Check sheet for the modelled part. Datum: model origin and axes. Units: mm. A direction names the side the tool comes from. Round coordinates to 2 decimals unless told otherwise and drop trailing zeros. Loops run counter-clockwise (first coordinate to the right, second up) from the corner with the lowest first, then second, coordinate; pieces in that order, holes last. Notation, with made-up numbers: (-26.5, -21.75) - (-5.5, -21.75) arc R5 cw to (-5.5, -14.75) - close; hole circle Ø9 at (2.5, 68.5). An arc over 180 degrees is marked (long way). Return JSON: item names as keys, results as strings.
from build123d import *

# Parameters (mm, degrees)
SKETCH1_R                = 6.985
BLANK_DISK_DEPTH         = 2
GEAR_TOOTH_CUT_DEPTH     = 11.657412937
GEAR_START               = -2.000000064
GEAR_TEETH_REVOLVE_DEPTH = 4.000000128
SKETCH4_R                = 0.75
HUB_EXTRUDE_DEPTH        = 0.635
HEX_BORE_CUT_DEPTH       = 11.643895353
HEX_BORE_CUT_DEPTH_BACK  = 11.643895353


# Read off the part's stored shape, not the designer's step: GEAR TEETH REVOLVE
with BuildPart() as part:
    # Sketch1 → BLANK DISK (new, symmetric)
    with BuildSketch(Plane.XY):
        Circle(SKETCH1_R)
    extrude(amount=BLANK_DISK_DEPTH, both=True)

    # Sketch2 → GEAR TOOTH CUT (cut, through all)
    with BuildSketch(Plane.XY.offset(2.000000064)):
        with BuildLine():
            ThreePointArc((-5.763009467, -3.946890786), (-6.563752956, -2.389010701), (-6.951733872, -0.680897326))
            ThreePointArc((-6.951733872, -0.680897326), (-6.303106227, -0.89616004), (-5.627259472, -0.997585))
            ThreePointArc((-5.627259472, -0.997585), (-5.00805343, -1.01182167), (-4.389706578, -0.976241119))
            ThreePointArc((-4.389706578, -0.976241119), (-4.103194142, -1.046520353), (-3.923782009, -1.280699416))
            ThreePointArc((-3.923782009, -1.280699416), (-3.878581292, -1.411688142), (-3.82900912, -1.541085788))
            ThreePointArc((-3.82900912, -1.541085788), (-3.815919388, -1.835801253), (-3.990226026, -2.073804914))
            ThreePointArc((-3.990226026, -2.073804914), (-4.486777934, -2.444014326), (-4.951966126, -2.852938219))
            ThreePointArc((-4.951966126, -2.852938219), (-5.404500069, -3.365060167), (-5.763009467, -3.946890786))
        make_face()
    extrude(amount=-GEAR_TOOTH_CUT_DEPTH, mode=Mode.SUBTRACT)

    # GEAR TEETH REVOLVE outline → GEAR TEETH REVOLVE (cut)
    with BuildSketch(Plane.XY.offset(GEAR_START)):
        with BuildLine():
            ThreePointArc((-4.887664738, -4.990086011), (-3.4925, -6.049187445), (-1.877708884, -6.727884834))
            ThreePointArc((-1.877708884, -6.727884834), (-1.977068265, -6.051731323), (-1.959592795, -5.368539939))
            ThreePointArc((-1.959592795, -5.368539939), (-1.866089177, -4.756268856), (-1.723674371, -4.15349458))
            ThreePointArc((-1.723674371, -4.15349458), (-1.743133543, -3.859131051), (-1.942600309, -3.641779824))
            ThreePointArc((-1.942600309, -3.641779824), (-2.06375, -3.574519854), (-2.182573688, -3.503231129))
            ThreePointArc((-2.182573688, -3.503231129), (-2.470538755, -3.439163456), (-2.735194635, -3.569493083))
            ThreePointArc((-2.735194635, -3.569493083), (-3.186005068, -3.994215061), (-3.669495571, -4.381327111))
            ThreePointArc((-3.669495571, -4.381327111), (-4.25241893, -4.738057004), (-4.887664738, -4.990086011))
        make_face()
        with BuildLine():
            ThreePointArc((-0.536602953, -6.964357994), (1.212932521, -6.878882154), (2.886192555, -6.360826796))
            ThreePointArc((2.886192555, -6.360826796), (2.375455753, -5.906730136), (1.949695784, -5.372142157))
            ThreePointArc((1.949695784, -5.372142157), (1.627763445, -4.843012329), (1.34940368, -4.289717971))
            ThreePointArc((1.34940368, -4.289717971), (1.14528386, -4.07673054), (0.852772776, -4.038444607))
            ThreePointArc((0.852772776, -4.038444607), (0.716732854, -4.064794001), (0.579885119, -4.086562064))
            ThreePointArc((0.579885119, -4.086562064), (0.318109172, -4.222583755), (0.199145275, -4.492539562))
            ThreePointArc((0.199145275, -4.492539562), (0.126810473, -5.107670834), (0.00526609, -5.714997574))
            ThreePointArc((0.00526609, -5.714997574), (-0.211977555, -6.362964438), (-0.536602953, -6.964357994))
        make_face()
        with BuildLine():
            ThreePointArc((4.065541317, -5.67992947), (5.350820435, -4.489871453), (6.29961242, -3.017467208))
            ThreePointArc((6.29961242, -3.017467208), (5.616477625, -2.997904272), (4.946700037, -2.862059354))
            ThreePointArc((4.946700037, -2.862059354), (4.35996746, -2.663656509), (3.791080751, -2.418734649))
            ThreePointArc((3.791080751, -2.418734649), (3.497810216, -2.386782502), (3.249124002, -2.545476276))
            ThreePointArc((3.249124002, -2.545476276), (3.161848439, -2.653105859), (3.071009233, -2.757745191))
            ThreePointArc((3.071009233, -2.757745191), (2.957910282, -3.030210187), (3.040302898, -3.313476852))
            ThreePointArc((3.040302898, -3.313476852), (3.380289985, -3.831190659), (3.677563689, -4.374557157))
            ThreePointArc((3.677563689, -4.374557157), (3.927650474, -5.010570096), (4.065541317, -5.67992947))
        make_face()
        with BuildLine():
            ThreePointArc((6.765373622, -1.737798823), (6.985, 0), (6.765373622, 1.737798823))
            ThreePointArc((6.765373622, 1.737798823), (6.229487195, 1.313674319), (5.629088366, 0.987212828))
            ThreePointArc((5.629088366, 0.987212828), (5.052094245, 0.762053795), (4.458869006, 0.584001497))
            ThreePointArc((4.458869006, 0.584001497), (4.213672298, 0.419967595), (4.125173997, 0.138548695))
            ThreePointArc((4.125173997, 0.138548695), (4.1275, 0), (4.125173997, -0.138548695))
            ThreePointArc((4.125173997, -0.138548695), (4.213672298, -0.419967595), (4.458869006, -0.584001497))
            ThreePointArc((4.458869006, -0.584001497), (5.052094245, -0.762053795), (5.629088366, -0.987212828))
            ThreePointArc((5.629088366, -0.987212828), (6.229487195, -1.313674319), (6.765373622, -1.737798823))
        make_face()
        with BuildLine():
            ThreePointArc((6.29961242, 3.017467208), (5.350820435, 4.489871453), (4.065541318, 5.679929471))
            ThreePointArc((4.065541318, 5.679929471), (3.927650474, 5.010570096), (3.677563689, 4.374557157))
            ThreePointArc((3.677563689, 4.374557157), (3.380289985, 3.831190659), (3.040302898, 3.313476852))
            ThreePointArc((3.040302898, 3.313476852), (2.957910282, 3.030210187), (3.071009233, 2.757745191))
            ThreePointArc((3.071009233, 2.757745191), (3.161848439, 2.653105859), (3.249124002, 2.545476276))
            ThreePointArc((3.249124002, 2.545476276), (3.497810216, 2.386782502), (3.791080751, 2.418734649))
            ThreePointArc((3.791080751, 2.418734649), (4.35996746, 2.663656509), (4.946700037, 2.862059354))
            ThreePointArc((4.946700037, 2.862059354), (5.616477625, 2.997904272), (6.29961242, 3.017467208))
        make_face()
        with BuildLine():
            ThreePointArc((2.886192555, 6.360826797), (1.212932521, 6.878882155), (-0.536602953, 6.964357994))
            ThreePointArc((-0.536602953, 6.964357994), (-0.211977555, 6.362964438), (0.00526609, 5.714997574))
            ThreePointArc((0.00526609, 5.714997574), (0.126810473, 5.107670834), (0.199145275, 4.492539562))
            ThreePointArc((0.199145275, 4.492539562), (0.318109172, 4.222583755), (0.579885119, 4.086562064))
            ThreePointArc((0.579885119, 4.086562064), (0.716732854, 4.064794001), (0.852772776, 4.038444607))
            ThreePointArc((0.852772776, 4.038444607), (1.14528386, 4.07673054), (1.34940368, 4.289717971))
            ThreePointArc((1.34940368, 4.289717971), (1.627763445, 4.843012329), (1.949695784, 5.372142157))
            ThreePointArc((1.949695784, 5.372142157), (2.375455753, 5.906730136), (2.886192555, 6.360826797))
        make_face()
        with BuildLine():
            ThreePointArc((-1.877708884, 6.727884835), (-3.4925, 6.049187445), (-4.887664739, 4.990086012))
            ThreePointArc((-4.887664739, 4.990086012), (-4.25241893, 4.738057004), (-3.669495571, 4.381327111))
            ThreePointArc((-3.669495571, 4.381327111), (-3.186005068, 3.994215061), (-2.735194635, 3.569493083))
            ThreePointArc((-2.735194635, 3.569493083), (-2.470538755, 3.439163456), (-2.182573688, 3.503231129))
            ThreePointArc((-2.182573688, 3.503231129), (-2.06375, 3.574519854), (-1.942600309, 3.641779824))
            ThreePointArc((-1.942600309, 3.641779824), (-1.743133543, 3.859131051), (-1.723674371, 4.15349458))
            ThreePointArc((-1.723674371, 4.15349458), (-1.866089177, 4.756268856), (-1.959592795, 5.368539939))
            ThreePointArc((-1.959592795, 5.368539939), (-1.977068265, 6.051731323), (-1.877708884, 6.727884835))
        make_face()
        with BuildLine():
            ThreePointArc((-3.923782009, 1.280699416), (-3.878581292, 1.411688142), (-3.82900912, 1.541085788))
            ThreePointArc((-3.82900912, 1.541085788), (-3.815919388, 1.835801253), (-3.990226026, 2.073804914))
            ThreePointArc((-3.990226026, 2.073804914), (-4.486777933, 2.444014326), (-4.951966126, 2.852938219))
            ThreePointArc((-4.951966126, 2.852938219), (-5.404500069, 3.365060167), (-5.763009467, 3.946890786))
            ThreePointArc((-5.763009467, 3.946890786), (-6.563752956, 2.389010701), (-6.951733872, 0.680897326))
            ThreePointArc((-6.951733872, 0.680897326), (-6.303106227, 0.89616004), (-5.627259472, 0.997585))
            ThreePointArc((-5.627259472, 0.997585), (-5.00805343, 1.01182167), (-4.389706578, 0.976241119))
            ThreePointArc((-4.389706578, 0.976241119), (-4.103194142, 1.046520353), (-3.923782009, 1.280699416))
        make_face()
    extrude(amount=GEAR_TEETH_REVOLVE_DEPTH, mode=Mode.SUBTRACT)

    # Sketch4 → Hub Extrude (add)
    with BuildSketch(Plane.XY.offset(2.000000064)):
        Circle(SKETCH4_R)
    extrude(amount=HUB_EXTRUDE_DEPTH)

    # Sketch3 → HEX BORE CUT (cut, two sides: drawn at the far end of the back side and taken through both)
    with BuildSketch(Plane.XY.offset(2.000000064).offset(-HEX_BORE_CUT_DEPTH_BACK)):
        with BuildLine():
            Line((-1.168931136, -0.94), (1.168931136, -0.94))
            ThreePointArc((1.168931136, -0.94), (0, 1.5), (-1.168931136, -0.94))
        make_face()
    extrude(amount=HEX_BORE_CUT_DEPTH + HEX_BORE_CUT_DEPTH_BACK, mode=Mode.SUBTRACT)


solid = part.part
Q1. Draft check along X on faces 1 (the face through (0.125, 5.116, -0.028)), 2 (the face through (3.501, 6.044, 0.028)), 3 (the face through (-1.978, 6.042, -0.028)). Enter one of: released by +X, released by -X, zero draft, split by the parting line, or undercut.
Answer key:
{"face 1": "undercut", "face 2": "released by +X", "face 3": "released by -X"}
Q2. Sectioned sample at B-B (x = 1.75). Enter the section's corners in (y, z), plus the area to 3 significant figures.
Answer key:
{"outline": "(-5.06, -2) - (5.06, -2) - (5.06, 2) - (-5.06, 2) - close", "area": "40.4 mm²"}
Q3. Depth check by flat-ended pin: P1, Ø1, axis at y = -4.5, z = 0.5, coming from the +X side; P2, Ø0.7, axis at x = 0, z = 1, coming from the +Y side; P3, Ø1.5, axis at x = 4.5, z = -0.5, coming from the -Y side. Enter the tip coordinate at first touch or a pass-through.
Answer key:
{"P1": "stops at x = 3.92", "P2": "stops at y = 6.65", "P3": "stops at y = -5.89"}
Q4. Scan lines: probe 1 along X at (y, z) = (0, 0.5) (1 decimal); probe 2 along Y at (x, z) = (3.25, 1); probe 3 along Y at (x, z) = (-0.25, 0.05). Record each from-to range of solid material in increasing order. Write a range as [from, to].
Answer key:
{"probe 1": "x = [-7, -1.5], [1.5, 4.1]", "probe 2": "y = [-6.18, -3.62], [-2.54, 2.54], [3.62, 6.18]", "probe 3": "y = [-6.45, -0.94], [1.48, 6.45]"}
Q5. Tool access check on faces 4 (the face through (-4.48, 2.44, -0.03)), 5 (the face through (-1.868, -4.765, -0.028)), 6 (the face through (5.04, -0.76, -0.03)), 7 (the face through (2.37, 5.9, -0.03)). Record the directions out of +Z, -Z, +X, -X, +Y, -Y that give a thin tool (end or side, any length) a straight path to the whole face; none if there is none.
Answer key:
{"face 4": "+Z, -Z, -X", "face 5": "+Z, -Z", "face 6": "+Z, -Z, +X", "face 7": "+Z, -Z, +Y"}
Q6. Sectioned sample at A-A (x = -1). Enter the section's corners in (y, z).
Answer key:
{"outline": "(-6.91, -2) - (-0.94, -2) - (-0.94, 2) - (-6.91, 2) - close; (1.12, -2) - (6.91, -2) - (6.91, 2) - (1.12, 2) - close"}
